Answer from the drawing. Dimensions are ordinates in mm from the lowest x, y and z of the part. Coordinates: 2 decimals unless noted, no trailing zeros. Write each loop counter-clockwise with the first axis right and the second up, starting at its lowest first coordinate (ties: lowest second). Pieces come first, ordered by that corner, then holes. Notation, with made-up numbers: (15.5, -10.75) -> (57.5, -10.75) arc R30 cw to (57.5, 27.25) -> close; hole circle Ø10 at (50.5, -37). An arc over 180 degrees is marked (long way). Use CSV: the item, a comma, the result in double quotes.
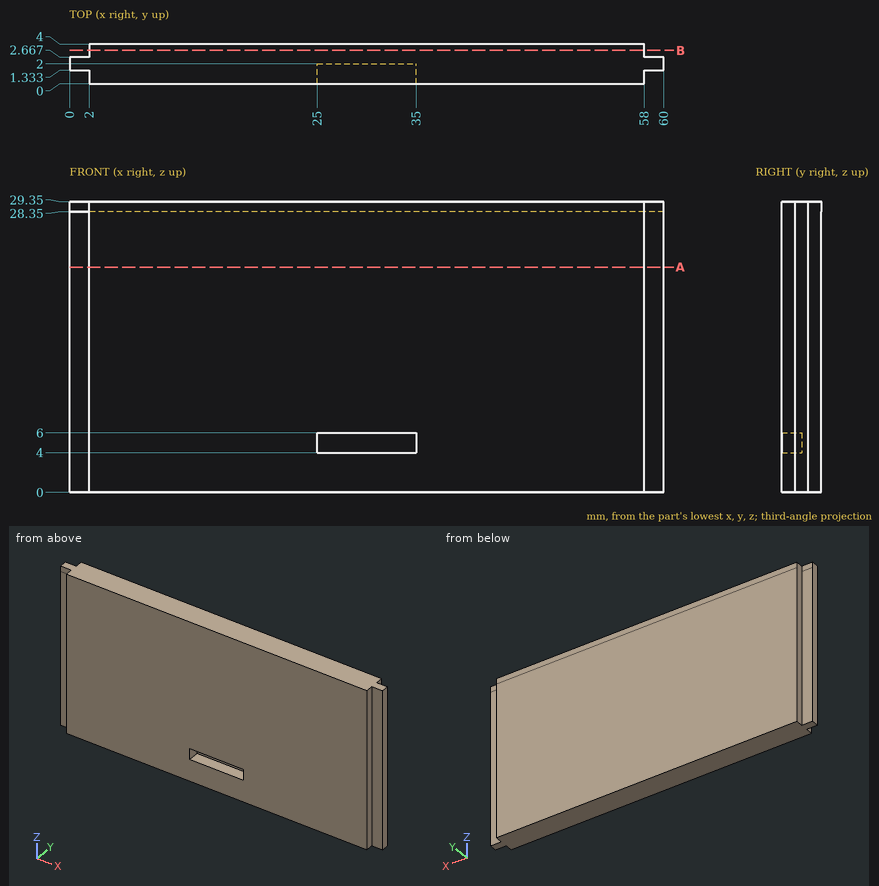
1. Find the intervals of material crossed by line 1 along X through (y, z) = (1.55, 5.5); line 2 along Z through (x, y) = (32, 1.2); line 3 along X through (y, z) = (2.95, 22.5), in increasing order.
Solutions:
line 1,"x = 0 to 25, 35 to 60"
line 2,"z = 0 to 4, 6 to 29.35"
line 3,"x = 2 to 58"
2. A cutting plane is placed at B-B (y = 3.35). Give the vertices of the cut face in (x, z).
Solutions:
outline,"(2, 0) -> (58, 0) -> (58, 29.35) -> (2, 29.35) -> close"
3. Each of these flat-tipped pins is pushed along its axis until it touches: pin 1 Ø0.6 at (y, z) = (1, 5) entering from -X; pin 2 Ø1.6 at (x, z) = (59, 13.5) entering from -Y; pin 3 Ø0.6 at (x, z) = (29.5, 5) entering from -Y. Where does it stop, or does it pass through?
Solutions:
pin 1,"stops at x = 2"
pin 2,"stops at y = 1.33"
pin 3,"stops at y = 2"
4. A cutting plane is placed at A-A (z = 22.75). Give the vertices of the cut face in (x, y), and give its area (3 significant figures).
Solutions:
outline,"(0, 1.33) -> (2, 1.33) -> (2, 0) -> (58, 0) -> (58, 1.33) -> (60, 1.33) -> (60, 2.67) -> (58, 2.67) -> (58, 4) -> (2, 4) -> (2, 2.67) -> (0, 2.67) -> close"
area,"229 mm^2"
